```python
from build123d import *

# Parameters (mm, degrees)
SKETCH1_W               = 30
SKETCH1_H               = 12.7
BOSS_EXTRUDE1_DEPTH     = 10
SKETCH2_R               = 8.2
CUT_EXTRUDE1_DEPTH      = 3.8
CUT_EXTRUDE2_START      = -3.1
SKETCH3_R               = 8.2
CUT_EXTRUDE2_DEPTH      = 3.1
CUT_EXTRUDE3_DEPTH      = 21.424495098
CUT_EXTRUDE3_DEPTH_BACK = 21.424495098
SKETCH4_R               = 6.2
FILLET1_R               = 2
SKETCH5_R               = 1.65
CUT_EXTRUDE4_DEPTH      = 20.113411522


with BuildPart() as part:
    # Sketch1 → Boss-Extrude1 (new body)
    with BuildSketch(Plane(origin=(0, 0, 0), x_dir=(1, 0, 0), z_dir=(0, 1, 0))):
        Rectangle(SKETCH1_W, SKETCH1_H)
    extrude(amount=BOSS_EXTRUDE1_DEPTH)

    # Sketch2 → Cut-Extrude1 (cut)
    with BuildSketch(Plane(origin=(0, 0, -6.35), x_dir=(-1, 0, 0), z_dir=(0, 0, -1))):
        with Locations((0, -0.55)):
            Circle(SKETCH2_R)
    extrude(amount=-CUT_EXTRUDE1_DEPTH, mode=Mode.SUBTRACT)

    # Sketch3 → Cut-Extrude2 (cut)
    with BuildSketch(Plane.XY.offset(6.35).offset(CUT_EXTRUDE2_START)):
        with Locations((0, -0.55)):
            Circle(SKETCH3_R)
    extrude(amount=CUT_EXTRUDE2_DEPTH, mode=Mode.SUBTRACT)

    # Sketch4 → Cut-Extrude3 (cut, two sides: drawn at the far end of the back side and taken through both)
    with BuildSketch(Plane.XY.offset(3.25).offset(-CUT_EXTRUDE3_DEPTH_BACK)):
        with Locations((0, -0.55)):
            Circle(SKETCH4_R)
    extrude(amount=CUT_EXTRUDE3_DEPTH + CUT_EXTRUDE3_DEPTH_BACK, mode=Mode.SUBTRACT)

    # Fillet1
    fillet1_edges = [part.edges().sort_by_distance(p)[0] for p in [
        (15, 5, 6.35),
        (-15, 5, 6.35),
        (-15, 5, -6.35),
        (15, 5, -6.35),
    ]]
    fillet(fillet1_edges, radius=FILLET1_R)

    # Sketch5 → Cut-Extrude4 (cut, symmetric)
    with BuildSketch(Plane.XZ):
        with Locations(Location((-11.590767043, 0, 0), (0, 0, 270))):
            Circle(SKETCH5_R)
    cut_extrude4 = extrude(amount=CUT_EXTRUDE4_DEPTH, both=True, mode=Mode.SUBTRACT)

    # Mirror1: Cut-Extrude4 across plane
    add(cut_extrude4.mirror(Plane(origin=(0, 0, 0), x_dir=(0, 0, 1), z_dir=(1, 0, 0))), mode=Mode.SUBTRACT)


solid = part.part
```
Read the model definition and answer for the solid it produces. Units are mm, in the model's axes. A direction names the side the tool comes from. Give positions to 0.01 mm unless a question says otherwise; leave off trailing zeros. Write each loop counter-clockwise with the first axis right and the second up, starting at its lowest first coordinate (ties: lowest second). Pieces come first, ordered by that corner, then holes. Notation, with made-up numbers: M 75.25,1.25 L 126.25,1.25 A28 cw 126.25,25.25 Z; hole C 62.5,7.25 d2. An arc over 180 degrees is marked long. Put each result on its own line as item: value. Start each with the question number.
1. The part is cut by section D-D, the plane y = 6. Give the vertices of the cut face in (x, z), and give its area (3 significant figures).
2. Which of the six approach directions +Z, -Z, +X, -X, +Y, -Y give full straight-line access (tool end or side, diameter ignored) to faces 1 (the cylindrical face through (-0.17, 7.65, -4.48)), 2 (the cylindrical face through (-13.2, 4.93, 0.36)), 3 (the flat face through (-1, 6, 3.25))?
3. For a pull along X with two mould halves and no side action, classify faces 4 (the flat face through (-15, 5, 0)), 5 (the cylindrical face through (14.4, 5.07, 5.78)), 6 (the flat face through (1, 6, -2.55)), 7 (the flat face through (0, 8, -6.35)) as released by +X, released by -X, zero draft, split by the parting line, or undercut.
4. Each of these flat-tipped pins is pushed along its axis until it touches: pin 1 Ø2 at (x, z) = (-11.59, 0) entering from +Y; pin 2 Ø4.5 at (x, z) = (11.59, 0) entering from -Y; pin 3 Ø4 at (x, y) = (-1, 5.5) entering from -Z; pin 4 Ø2 at (x, y) = (-4, 5) entering from +Z. Where does it stop, or does it pass through?
5. Consider line 1 along X through (y, z) = (7.5, 0); line 2 along X through (y, z) = (7, -1.5); line 3 along X through (y, z) = (3, 0). Determine where each line is inside the solid, lowest interval first.
6. The part is cut by section A-A, the plane z = 0. Give the vertices of the cut face in (x, y).
7. The part is cut by section C-C, the plane x = -11. Give the vertices of the cut face in (y, z), and give its area (3 significant figures).
8. The part is cut by section B-B, the plane y = 4. Give the vertices of the cut face in (x, z).
Final values:
1. outline: M -15,-4.35 A2 ccw -13,-6.35 L -4.93,-6.35 L -4.93,-2.55 L 4.93,-2.55 L 4.93,-6.35 L 13,-6.35 A2 ccw 15,-4.35 L 15,4.35 A2 ccw 13,6.35 L 4.93,6.35 L 4.93,3.25 L -4.93,3.25 L -4.93,6.35 L -13,6.35 A2 ccw -15,4.35 Z; hole C -11.59,0 d3.3; hole C 11.59,0 d3.3
1. area: 292 mm²
2. face 1: -Z, -Y
2. face 2: +Y, -Y
2. face 3: +Z, -Y
3. face 4: released by -X
3. face 5: released by +X
3. face 6: undercut
3. face 7: zero draft
4. pin 1: passes through
4. pin 2: stops at y = 0
4. pin 3: stops at z = -2.55
4. pin 4: stops at z = 3.25
5. line 1: x = -15 to -13.24, -9.94 to 9.94, 13.24 to 15
5. line 2: x = -15 to -12.28, -10.9 to 10.9, 12.28 to 15
5. line 3: x = -15 to -13.24, -9.94 to -5.08, 5.08 to 9.94, 13.24 to 15
6. outline: M -15,0 L -13.24,0 L -13.24,10 L -15,10 Z; M -9.94,0 L -6.18,0 A6.2 cw 6.18,0 L 9.94,0 L 9.94,10 L -9.94,10 Z; M 13.24,0 L 15,0 L 15,10 L 13.24,10 Z
7. outline: M 0,-6.35 L 10,-6.35 L 10,-1.54 L 0,-1.54 Z; M 0,1.54 L 10,1.54 L 10,6.35 L 0,6.35 Z
7. area: 96.2 mm²
8. outline: M -15,-4.35 A2 ccw -13,-6.35 L -6.82,-6.35 L -6.82,-2.55 L -4.21,-2.55 L -4.21,3.25 L -6.82,3.25 L -6.82,6.35 L -13,6.35 A2 ccw -15,4.35 Z; M 4.21,-2.55 L 6.82,-2.55 L 6.82,-6.35 L 13,-6.35 A2 ccw 15,-4.35 L 15,4.35 A2 ccw 13,6.35 L 6.82,6.35 L 6.82,3.25 L 4.21,3.25 Z; hole C -11.59,0 d3.3; hole C 11.59,0 d3.3
